```python
from build123d import *

# Parameters (mm, degrees)
SKETCH1_W           = 2.5
SKETCH1_H           = 17
BOSS_EXTRUDE1_DEPTH = 100
SKETCH1_3_W         = 2.5
SKETCH1_3_H         = 12
BOSS_EXTRUDE2_DEPTH = 3


with BuildPart() as part:
    # Sketch1 → Boss-Extrude1 (new body)
    with BuildSketch(Plane.XY):
        Rectangle(SKETCH1_W, SKETCH1_H)
    extrude(amount=BOSS_EXTRUDE1_DEPTH)

    # Sketch1<3> → Boss-Extrude2 (add)
    with BuildSketch(Plane.XY):
        Rectangle(SKETCH1_3_W, SKETCH1_3_H)
    boss_extrude2 = extrude(amount=-BOSS_EXTRUDE2_DEPTH)

    # Mirror1: Boss-Extrude2 across plane
    add(boss_extrude2.mirror(Plane(origin=(0, 0, 50), x_dir=(1, 0, 0), z_dir=(0, 0, -1))))


solid = part.part
```
The model under review builds one solid part; all positions refer to its coordinate system, in mm. A direction names the side the tool comes from. Round coordinates to 2 decimals unless told otherwise and drop trailing zeros. Write each loop counter-clockwise with the first axis right and the second up, starting at its lowest first coordinate (ties: lowest second). Pieces come first, ordered by that corner, then holes. Notation, with made-up numbers: (58, 68.5) - (65, 68.5) arc R7 cw to (65, 75.5) - close; hole circle Ø3 at (4.5, 5). An arc over 180 degrees is marked (long way). Answer as CSV lines item,"result". Start each with the question number.
(1) To check wall thickness, follow line 1 (Z direction, x = 1, y = 7). State the ranges of the line that lie inside material, in increasing order.
(2) For faces 1 (the flat face through (0, -6, 101)), 2 (the flat face through (0, 6, 101)), 3 (the flat face through (0, -7, 0)), list the 3-axis set-ups (+Z, -Z, +X, -X, +Y, -Y) from which the entire face can be reached by the end or side of a thin tool; tool diameter is ignored.
(3) We need section A-A on x = -0.2. State the section outline as (y, z) points, plus the area to 3 significant figures.
(4) For pin 1 Ø0.8 at (x, y) = (-0.5, -7.5) entering from +Z; pin 2 Ø1.2 at (x, z) = (0.5, -1.5) entering from +Y; pin 3 Ø0.8 at (x, z) = (-0.5, -2) entering from -Y, all flat-tipped, find the tip position at first contact; note any pin that passes through.
Worked answers:
1,line 1,"0 to 100"
2,face 1,"+Z, +X, -X, -Y"
2,face 2,"+Z, +X, -X, +Y"
2,face 3,"-Z, +X, -X, -Y"
3,outline,"(-8.5, 0) - (-6, 0) - (-6, -3) - (6, -3) - (6, 0) - (8.5, 0) - (8.5, 100) - (6, 100) - (6, 103) - (-6, 103) - (-6, 100) - (-8.5, 100) - close"
3,area,"1,770 mm²"
4,pin 1,"z = 100"
4,pin 2,"y = 6"
4,pin 3,"y = -6"
